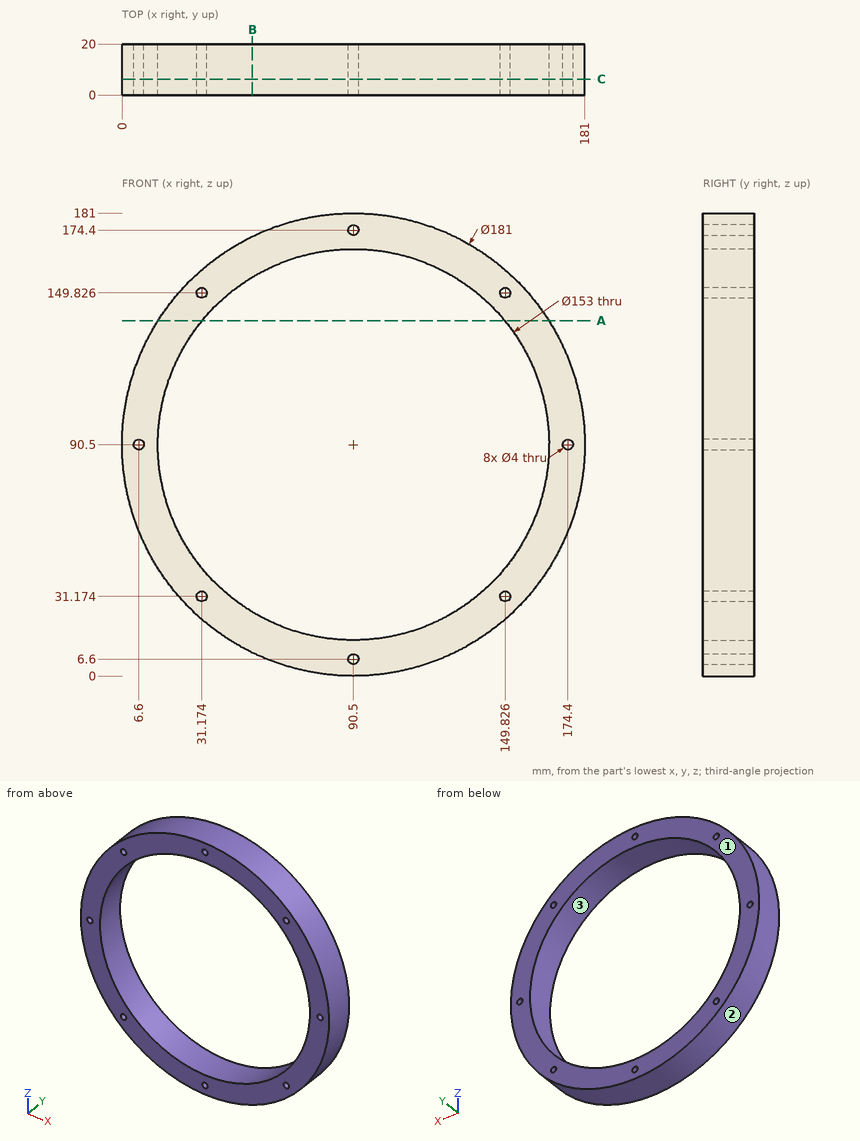
Geometry: see drawing. Coordinates: mm, zero at the bounding-box minimum. Coordinates: 2 decimals unless noted, no trailing zeros. Loops run counter-clockwise (first coordinate to the right, second up) from the corner with the lowest first, then second, coordinate; pieces in that order, holes last. Notation, with made-up numbers: M 81,33.5 L 90,33.5 A12 ccw 90,38.5 Z; hole C -8,-22 d1. An arc over 180 degrees is marked long. Put each result on its own line as item: value. Start each with the question number.
1) Cut plane A-A on z = 139. Return the cut outline in (x, y), then the cut area to 3 significant figures.
2) Ray query, L1, parallel to Z at x = 113, y = 4; L2, parallel to Z at x = 55.5, y = 16.25; L3, parallel to X at y = 14.75, z = 54. Return the intervals inside material, ascending. Write a range as from..to.
3) Contact query for flat-ended pins moving along their axis: pin 1 Ø1 at (x, y) = (61.5, 15) entering from -Z (1 decimal); pin 2 Ø4 at (x, y) = (54, 10.5) entering from -Z; pin 3 Ø3 at (x, y) = (29.5, 12.5) entering from -Z. Output: stop coordinate, or through.
4) Cut plane C-C on y = 6.25. Give the number of separate pieces and of enclosed holes in the cut face.
5) Cut plane B-B on x = 51. Return the cut outline in (y, z) (1 decimal).
6) Pull-direction query (Z, two-part tool) for the marked faces 1, 2 and 3; classes: pulls with the +Z half, pulls with the -Z half, needs draft (parallel to the pull), parting line crosses it, or undercut.
The answers:
1. outline: M 14.09,0 L 31.34,0 L 31.34,20 L 14.09,20 Z; M 149.66,0 L 166.91,0 L 166.91,20 L 149.66,20 Z
1. area: 690 mm²
2. L1: z = 2.84..17.38, 163.62..178.16
2. L2: z = 7.04..22.48, 158.52..173.96
2. L3: x = 7.69..23.27, 157.73..173.31
3. pin 1: stops at z = 4.6
3. pin 2: stops at z = 6.83
3. pin 3: stops at z = 22.31
4. separate pieces: 1
4. enclosed holes: 9
5. outline: M 0,9.1 L 20,9.1 L 20,25 L 0,25 Z; M 0,156 L 20,156 L 20,171.9 L 0,171.9 Z
6. face 1: needs draft
6. face 2: parting line crosses it
6. face 3: undercut
